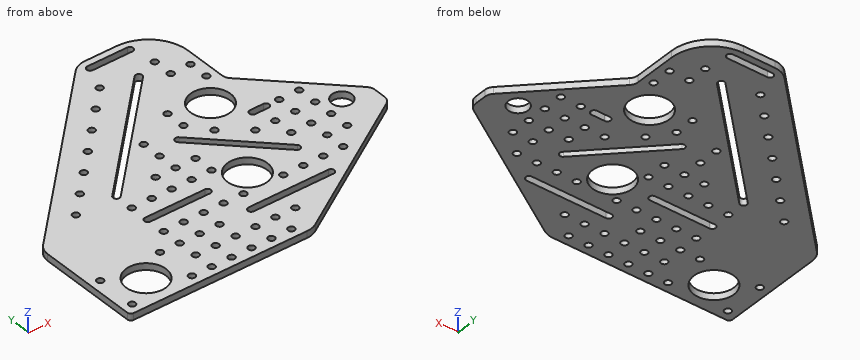
from build123d import *

# Parameters (mm, degrees)
MODEL_R                 = 1.5
MODEL_R_2               = 9
MODEL_R_3               = 4.5
SALIENTE_EXTRUIR1_DEPTH = 3


with BuildPart() as part:
    # Model → Saliente-Extruir1 (new body)
    with BuildSketch(Plane.XY):
        with BuildLine():
            Line((-523.445769407, 701.09903587), (-509.173691468, 701.09903587))
            ThreePointArc((-509.173691468, 701.09903587), (-496.445769407, 695.826957932), (-491.173691468, 683.09903587))
            Line((-491.173691468, 683.09903587), (-491.173691468, 664.240109283))
            ThreePointArc((-491.173691468, 664.240109283), (-490.831149364, 662.518033837), (-489.855671983, 661.058128768))
            Line((-489.855671983, 661.058128768), (-455.785034404, 626.987491188))
            ThreePointArc((-455.785034404, 626.987491188), (-454.809557023, 625.527586118), (-454.467014919, 623.805510673))
            Line((-454.467014919, 623.805510673), (-454.467014919, 618.640217135))
            ThreePointArc((-454.467014919, 618.640217135), (-455.028739924, 616.463065312), (-456.573677169, 614.829451541))
            Line((-456.573677169, 614.829451541), (-521.120267881, 574.29119528))
            ThreePointArc((-521.120267881, 574.29119528), (-523.416339106, 573.264206922), (-525.906943381, 572.912726468))
            Line((-525.906943381, 572.912726468), (-604.315119618, 572.912726468))
            ThreePointArc((-604.315119618, 572.912726468), (-605.37577979, 573.352066296), (-605.815119618, 574.412726468))
            Line((-605.815119618, 574.412726468), (-605.815119618, 619.352823846))
            ThreePointArc((-605.815119618, 619.352823846), (-605.217350164, 622.286969974), (-603.519329352, 624.753397987))
            Line((-603.519329352, 624.753397987), (-529.809730437, 698.462996901))
            ThreePointArc((-529.809730437, 698.462996901), (-526.889920298, 700.413951663), (-523.445769407, 701.09903587))
        make_face()
        with Locations((-601.315119618, 595.412726468)):
            Circle(MODEL_R, mode=Mode.SUBTRACT)
        with Locations((-574.315119618, 577.412726468)):
            Circle(MODEL_R, mode=Mode.SUBTRACT)
        with Locations((-601.315119618, 577.412726468)):
            Circle(MODEL_R, mode=Mode.SUBTRACT)
        with Locations((-574.315119618, 595.412726468)):
            Circle(MODEL_R, mode=Mode.SUBTRACT)
        with Locations((-587.815119618, 586.412726468)):
            Circle(MODEL_R_2, mode=Mode.SUBTRACT)
        with Locations((-565.459568289, 586.351847961)):
            Circle(MODEL_R, mode=Mode.SUBTRACT)
        with Locations((-556.459568289, 586.351847961)):
            Circle(MODEL_R, mode=Mode.SUBTRACT)
        with Locations((-547.459568289, 586.351847961)):
            Circle(MODEL_R, mode=Mode.SUBTRACT)
        with Locations((-538.459568289, 586.351847961)):
            Circle(MODEL_R, mode=Mode.SUBTRACT)
        with Locations((-529.459568289, 586.351847961)):
            Circle(MODEL_R, mode=Mode.SUBTRACT)
        with Locations((-565.459568289, 595.351847961)):
            Circle(MODEL_R, mode=Mode.SUBTRACT)
        with Locations((-556.459568289, 595.351847961)):
            Circle(MODEL_R, mode=Mode.SUBTRACT)
        with Locations((-547.459568289, 595.351847961)):
            Circle(MODEL_R, mode=Mode.SUBTRACT)
        with Locations((-520.459568289, 586.351847961)):
            Circle(MODEL_R, mode=Mode.SUBTRACT)
        with Locations((-565.459568289, 604.351847961)):
            Circle(MODEL_R, mode=Mode.SUBTRACT)
        with Locations((-556.459568289, 604.351847961)):
            Circle(MODEL_R, mode=Mode.SUBTRACT)
        with Locations((-547.459568289, 604.351847961)):
            Circle(MODEL_R, mode=Mode.SUBTRACT)
        with Locations((-538.459568289, 604.351847961)):
            Circle(MODEL_R, mode=Mode.SUBTRACT)
        with Locations((-529.459568289, 604.351847961)):
            Circle(MODEL_R, mode=Mode.SUBTRACT)
        with Locations((-511.459568289, 604.351847961)):
            Circle(MODEL_R, mode=Mode.SUBTRACT)
        with Locations((-556.459568289, 622.351847961)):
            Circle(MODEL_R, mode=Mode.SUBTRACT)
        with Locations((-547.459568289, 622.351847961)):
            Circle(MODEL_R, mode=Mode.SUBTRACT)
        with Locations((-538.459568289, 622.351847961)):
            Circle(MODEL_R, mode=Mode.SUBTRACT)
        with Locations((-529.459568289, 622.351847961)):
            Circle(MODEL_R, mode=Mode.SUBTRACT)
        with Locations((-520.459568289, 613.351847961)):
            Circle(MODEL_R_2, mode=Mode.SUBTRACT)
        with Locations((-547.459568289, 631.351847961)):
            Circle(MODEL_R, mode=Mode.SUBTRACT)
        with Locations((-538.459568289, 631.351847961)):
            Circle(MODEL_R, mode=Mode.SUBTRACT)
        with Locations((-538.459568289, 640.351847961)):
            Circle(MODEL_R, mode=Mode.SUBTRACT)
        with Locations((-529.459568289, 631.351847961)):
            Circle(MODEL_R, mode=Mode.SUBTRACT)
        with Locations((-513.673691468, 640.351847961)):
            Circle(MODEL_R, mode=Mode.SUBTRACT)
        with Locations((-495.673691468, 667.351847961)):
            Circle(MODEL_R, mode=Mode.SUBTRACT)
        with Locations((-504.673691468, 653.851847961)):
            Circle(MODEL_R_2, mode=Mode.SUBTRACT)
        with Locations((-502.459568289, 604.351847961)):
            Circle(MODEL_R, mode=Mode.SUBTRACT)
        with Locations((-502.459568289, 631.351847961)):
            Circle(MODEL_R, mode=Mode.SUBTRACT)
        with Locations((-495.673691468, 676.351847961)):
            Circle(MODEL_R, mode=Mode.SUBTRACT)
        with Locations((-504.588556274, 685.351847961)):
            Circle(MODEL_R, mode=Mode.SUBTRACT)
        with Locations((-504.588556274, 676.351847961)):
            Circle(MODEL_R, mode=Mode.SUBTRACT)
        with Locations((-556.459568289, 658.351847961)):
            Circle(MODEL_R, mode=Mode.SUBTRACT)
        with Locations((-547.459568289, 667.351847961)):
            Circle(MODEL_R, mode=Mode.SUBTRACT)
        with Locations((-538.459568289, 676.351847961)):
            Circle(MODEL_R, mode=Mode.SUBTRACT)
        with Locations((-529.459568289, 685.351847961)):
            Circle(MODEL_R, mode=Mode.SUBTRACT)
        with Locations((-574.459568289, 640.351847961)):
            Circle(MODEL_R, mode=Mode.SUBTRACT)
        with Locations((-565.459568289, 649.351847961)):
            Circle(MODEL_R, mode=Mode.SUBTRACT)
        with Locations((-583.459568289, 631.351847961)):
            Circle(MODEL_R, mode=Mode.SUBTRACT)
        with Locations((-565.459568289, 622.351847961)):
            Circle(MODEL_R, mode=Mode.SUBTRACT)
        with Locations((-493.459568289, 631.351847961)):
            Circle(MODEL_R, mode=Mode.SUBTRACT)
        with Locations((-484.459568289, 631.351847961)):
            Circle(MODEL_R, mode=Mode.SUBTRACT)
        with Locations((-475.459568289, 631.351847961)):
            Circle(MODEL_R, mode=Mode.SUBTRACT)
        with Locations((-484.459568289, 613.351847961)):
            Circle(MODEL_R, mode=Mode.SUBTRACT)
        with Locations((-484.459568289, 622.351847961)):
            Circle(MODEL_R, mode=Mode.SUBTRACT)
        with Locations((-475.459568289, 613.351847961)):
            Circle(MODEL_R, mode=Mode.SUBTRACT)
        with Locations((-493.459568289, 622.351847961)):
            Circle(MODEL_R, mode=Mode.SUBTRACT)
        with Locations((-493.459568289, 604.351847961)):
            Circle(MODEL_R, mode=Mode.SUBTRACT)
        with Locations((-484.459568289, 604.351847961)):
            Circle(MODEL_R, mode=Mode.SUBTRACT)
        with Locations((-520.459568289, 649.351847961)):
            Circle(MODEL_R, mode=Mode.SUBTRACT)
        with Locations((-520.459568289, 658.351847961)):
            Circle(MODEL_R, mode=Mode.SUBTRACT)
        with Locations((-475.459568289, 622.351847961)):
            Circle(MODEL_R, mode=Mode.SUBTRACT)
        with Locations((-484.459568289, 640.351847961)):
            Circle(MODEL_R, mode=Mode.SUBTRACT)
        with Locations((-475.459568289, 640.351847961)):
            Circle(MODEL_R, mode=Mode.SUBTRACT)
        with Locations((-565.459568289, 577.351847961)):
            Circle(MODEL_R, mode=Mode.SUBTRACT)
        with Locations((-556.459568289, 577.351847961)):
            Circle(MODEL_R, mode=Mode.SUBTRACT)
        with Locations((-547.459568289, 577.351847961)):
            Circle(MODEL_R, mode=Mode.SUBTRACT)
        with Locations((-538.459568289, 577.351847961)):
            Circle(MODEL_R, mode=Mode.SUBTRACT)
        with Locations((-529.459568289, 577.351847961)):
            Circle(MODEL_R, mode=Mode.SUBTRACT)
        with Locations((-538.459568289, 649.351847961)):
            Circle(MODEL_R, mode=Mode.SUBTRACT)
        with Locations((-466.989899424, 626.851847961)):
            Circle(MODEL_R_3, mode=Mode.SUBTRACT)
        with BuildLine():
            Line((-515.506429579, 683.06781295), (-566.418117824, 632.156124705))
            ThreePointArc((-566.418117824, 632.156124705), (-566.418117824, 630.034804361), (-564.29679748, 630.034804361))
            Line((-564.29679748, 630.034804361), (-513.385109235, 680.946492606))
            ThreePointArc((-513.385109235, 680.946492606), (-513.385109235, 683.06781295), (-515.506429579, 683.06781295))
        make_face(mode=Mode.SUBTRACT)
        with BuildLine():
            Line((-496.414546486, 615.185561956), (-526.113031296, 644.884046766))
            ThreePointArc((-526.113031296, 644.884046766), (-528.23435164, 644.884046766), (-528.23435164, 642.762726422))
            Line((-528.23435164, 642.762726422), (-498.53586683, 613.064241613))
            ThreePointArc((-498.53586683, 613.064241613), (-496.414546486, 613.064241613), (-496.414546486, 615.185561956))
        make_face(mode=Mode.SUBTRACT)
        with BuildLine():
            Line((-506.763788891, 698.09903587), (-524.763788891, 698.09903587))
            ThreePointArc((-524.763788891, 698.09903587), (-526.263788891, 696.59903587), (-524.763788891, 695.09903587))
            Line((-524.763788891, 695.09903587), (-506.763788891, 695.09903587))
            ThreePointArc((-506.763788891, 695.09903587), (-505.263788891, 696.59903587), (-506.763788891, 698.09903587))
        make_face(mode=Mode.SUBTRACT)
        with BuildLine():
            Line((-565.459568289, 614.851847961), (-538.459568289, 614.851847961))
            ThreePointArc((-538.459568289, 614.851847961), (-536.959568289, 613.351847961), (-538.459568289, 611.851847961))
            Line((-538.459568289, 611.851847961), (-565.459568289, 611.851847961))
            ThreePointArc((-565.459568289, 611.851847961), (-566.959568289, 613.351847961), (-565.459568289, 614.851847961))
        make_face(mode=Mode.SUBTRACT)
        with BuildLine():
            Line((-496.459568289, 641.851847961), (-490.459568289, 641.851847961))
            ThreePointArc((-490.459568289, 641.851847961), (-488.959568289, 640.351847961), (-490.459568289, 638.851847961))
            Line((-490.459568289, 638.851847961), (-496.459568289, 638.851847961))
            ThreePointArc((-496.459568289, 638.851847961), (-497.959568289, 640.351847961), (-496.459568289, 641.851847961))
        make_face(mode=Mode.SUBTRACT)
        with BuildLine():
            Line((-533.170047289, 596.851847961), (-497.173691468, 596.851847961))
            ThreePointArc((-497.173691468, 596.851847961), (-495.673691468, 595.351847961), (-497.173691468, 593.851847961))
            Line((-497.173691468, 593.851847961), (-533.170047289, 593.851847961))
            ThreePointArc((-533.170047289, 593.851847961), (-534.670047289, 595.351847961), (-533.170047289, 596.851847961))
        make_face(mode=Mode.SUBTRACT)
    extrude(amount=SALIENTE_EXTRUIR1_DEPTH)


solid = part.part
Geometry: final body of the model. Coordinates: model frame, mm. Give positions to 0.01 mm unless a question says otherwise; leave off trailing zeros. Order: outer loops, then holes, each group sorted by start corner. A loop starts at its lowest first (then second) coordinate and runs counter-clockwise, first axis right, second up. Notation, with made-up numbers: (-13, 48) - (46, 48) arc R27 ccw to (46, 77) - close; hole circle Ø2 at (16, 89.5). An arc over 180 degrees is marked (long way). Use CSV: the item, a comma, the result in double quotes.
1. Section query A-A (x = -542.5). Output: boundary loops of the cut face in (y, z).
Answers below:
outline,"(572.91, 0) - (611.85, 0) - (611.85, 3) - (572.91, 3) - close; (614.85, 0) - (651.83, 0) - (651.83, 3) - (614.85, 3) - close; (656.07, 0) - (685.77, 0) - (685.77, 3) - (656.07, 3) - close"
2. Section query C-C (x = -561.5). Output: boundary loops of the cut face in (y, z).
Answers below:
outline,"(572.91, 0) - (611.85, 0) - (611.85, 3) - (572.91, 3) - close; (614.85, 0) - (632.83, 0) - (632.83, 3) - (614.85, 3) - close; (637.07, 0) - (666.77, 0) - (666.77, 3) - (637.07, 3) - close"
3. Section query B-B (y = 591.5). Output: boundary loops of the cut face in (x, z).
Answers below:
outline,"(-605.82, 0) - (-595.24, 0) - (-595.24, 3) - (-605.82, 3) - close; (-580.39, 0) - (-493.72, 0) - (-493.72, 3) - (-580.39, 3) - close"
4. Section query D-D (z = 2.05). Give the number of separate pieces and of enclosed holes in the cut face, plus the area to 3 significant figures.
Answers below:
separate pieces,"1"
enclosed holes,"72"
area,"10,700 mm2"
5. Material intervals for line 1 along Y through (x, z) = (-575.5, 0.45); line 2 along Y through (x, z) = (-533.5, 1.8); line 3 along X through (y, z) = (643.5, 0.85), sorted ascending. Write a range as from..to.
Answers below:
line 1,"572.91..576.49, 578.33..594.49, 596.33..639.27, 641.43..652.77"
line 2,"572.91..593.89, 596.82..660.83, 665.07..694.77"
line 3,"-584.77..-555.07, -550.83..-528.64, -524.73..-472.3"
6. Contact query for a flat-ended pin moving along its axis: pin 1 (2.5 mm diameter, centred on x = -538.46, y = 586.35, fed in from +Z). Output: stop coordinate, or through.
Answers below:
pin 1,"through"
